```python
from build123d import *

# Parameters (mm, degrees)
SKETCH3_R          = 2.38125
SKETCH3_R_2        = 9.525
CUT_EXTRUDE1_DEPTH = 31.700788874


with BuildPart() as part:
    # Sketch2 → Revolve1 (revolve)
    with BuildSketch(Plane.XY, mode=Mode.PRIVATE) as revolve1_sk:
        Polygon((0, 0), (0, 19.05), (0, 20.6375), (1.5875, 20.6375), (1.5875, 19.05), (7.9375, 19.05), (7.9375, 20.6375), (9.525, 20.6375), (9.525, 19.05), (9.525, 0), align=None)
    revolve(revolve1_sk.sketch.rotate(Axis((0, 0, 0), (1, 0, 0)), 90), axis=Axis((0, 0, 0), (1, 0, 0)))

    # Sketch3 → Cut-Extrude1 (cut, through all)
    with BuildSketch(Plane.ZY):
        with Locations((-12.7, 0)):
            Circle(SKETCH3_R)
        with Locations((6.858, 0)):
            Circle(SKETCH3_R_2)
    extrude(amount=-CUT_EXTRUDE1_DEPTH, mode=Mode.SUBTRACT)


solid = part.part
```
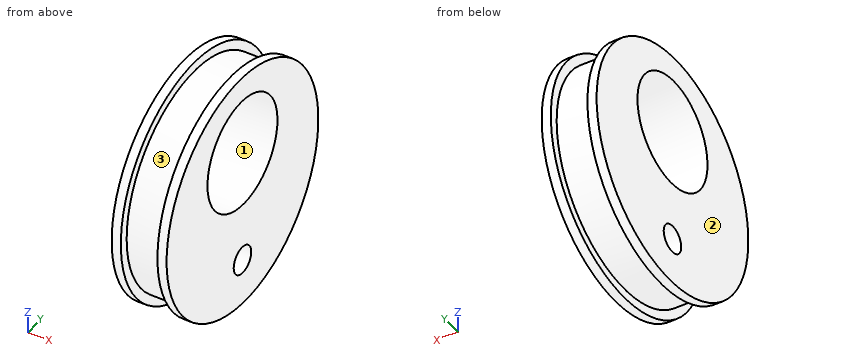
The listing builds one solid part. Answer for the finished solid, in the listing's coordinates (mm). Face numbers are marked on the shaded views. Give positions to 0.01 mm unless a question says otherwise; leave off trailing zeros. Loops run counter-clockwise (first coordinate to the right, second up) from the corner with the lowest first, then second, coordinate; pieces in that order, holes last. Notation, with made-up numbers: (-7.75, -10.5) - (5.25, -10.5) arc R38 cw to (5.25, 27.5) - close; hole circle Ø1 at (16, 36.5). An arc over 180 degrees is marked (long way). Answer as CSV lines item,"result". Start each with the question number.
Item 1: A cutting plane is placed at B-B on y = 0. Count the separate pieces of the cut face and the enclosed holes in it, then the cut area to 3 significant figures.
Item 2: Each of these flat-tipped pins is pushed along its axis until it touches: pin 1 (5.5 mm diameter, centred on y = 0, z = -12.7, fed in from -X); pin 2 (4 mm diameter, centred on y = -3, z = 1.5, fed in from -X); pin 3 (1 mm diameter, centred on x = 1, z = -2, fed in from +Y); pin 4 (2 mm diameter, centred on x = 6, z = 15, fed in from +Y). Where does it stop, or does it pass through?
Item 3: The mould has two halves that part along Z. Classify the marked faces 1, 2 and 3: +Z half, -Z half, draft (parallel to the pull), parting line (faces both ways), or undercut.
Item 4: Find the intervals of material crossed by line 1 (X direction, y = -10.5, z = 16) (1 decimal); line 2 (Z direction, x = 8.75, y = -0.5); line 3 (Z direction, x = 5, y = 2.5), in increasing order. Write a range as from..to.
Item 5: A cutting plane is placed at D-D on y = 5. Determine the outline of the cut face in (x, z) (1 decimal), then the cut area to 3 significant figures.
Found:
1,separate pieces,"3"
1,enclosed holes,"0"
1,area,"146 mm^2"
2,pin 1,"stops at x = 0"
2,pin 2,"passes through"
2,pin 3,"stops at y = 20.58"
2,pin 4,"stops at y = 12.92"
3,face 1,"undercut"
3,face 2,"draft"
3,face 3,"parting line"
4,line 1,"x = 0..1.6, 7.9..9.5"
4,line 2,"z = -20.63..-15.03, -10.37..-2.65, 16.37..20.63"
4,line 3,"z = -18.89..-2.33, 16.05..18.89"
5,outline,"(0, -20) - (1.6, -20) - (1.6, -18.4) - (7.9, -18.4) - (7.9, -20) - (9.5, -20) - (9.5, -1.2) - (0, -1.2) - close; (0, 15) - (9.5, 15) - (9.5, 20) - (7.9, 20) - (7.9, 18.4) - (1.6, 18.4) - (1.6, 20) - (0, 20) - close"
5,area,"206 mm^2"
